Source: CAD feature listing. Evaluate the final solid. Frame: model axes, mm. Face numbers are marked on the shaded views. A direction names the side the tool comes from. Coordinates: 2 decimals unless noted, no trailing zeros. Loops run counter-clockwise (first coordinate to the right, second up) from the corner with the lowest first, then second, coordinate; pieces in that order, holes last. Notation, with made-up numbers: (2, 64.25) -> (57, 64.25) arc R16 ccw to (57, 83.25) -> close; hole circle Ø7 at (63.25, 50.5). An arc over 180 degrees is marked (long way). Answer as CSV lines item,"result".
from build123d import *

# Parameters (mm, degrees)
SCHIZZO1_R                   = 35
ESTRUSIONE_ESTRUSIONE1_DEPTH = 20
SCHIZZO2_R                   = 15
ESTRUSIONE_ESTRUSIONE2_DEPTH = 30
RACCORDO1_R                  = 20


with BuildPart() as part:
    # Schizzo1 → Estrusione-Estrusione1 (new body)
    with BuildSketch(Plane(origin=(0, 0, 0), x_dir=(1, 0, 0), z_dir=(0, 1, 0))):
        with Locations(Location((0, 0, 0), (0, 0, 270))):
            Circle(SCHIZZO1_R)
    extrude(amount=ESTRUSIONE_ESTRUSIONE1_DEPTH)

    # Schizzo2 → Estrusione-Estrusione2 (add)
    with BuildSketch(Plane(origin=(0, 20, 0), x_dir=(1, 0, 0), z_dir=(0, 1, 0))):
        with Locations(Location((0, 0, 0), (0, 0, 270))):
            Circle(SCHIZZO2_R)
    extrude(amount=ESTRUSIONE_ESTRUSIONE2_DEPTH)

    # Raccordo1
    raccordo1_edges = [part.edges().sort_by_distance(p)[0] for p in [
        (0, 20, -15),
    ]]
    fillet(raccordo1_edges, radius=RACCORDO1_R - 0.0001)  # a hair under: the kernel refuses the full size

    # Smusso1: read off the stored shape, not the designer's step
    # Smusso1 outline → Smusso1 (revolve, cut)
    with BuildSketch(Plane.XY):
        Polygon((35, 21.143819168), (28.333333333, 21.143819168), (35, 11.715728753), align=None)
    revolve(axis=Axis((0, 0, 0), (0, 1, 0)), mode=Mode.SUBTRACT)


solid = part.part
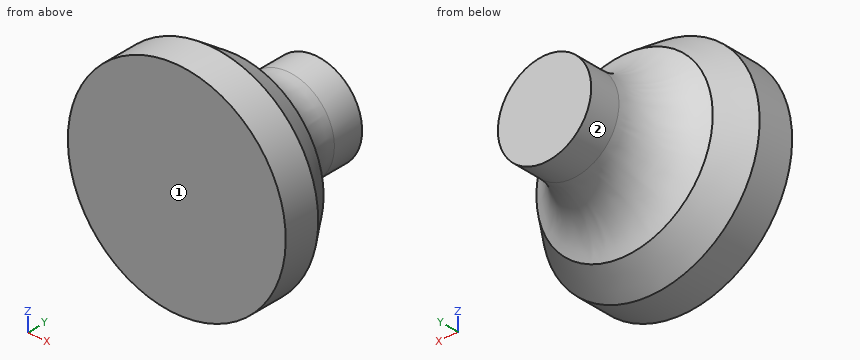
(1) Cut plane A-A (x = 0). Return the cut outline in (y, z).
Computed values:
outline,"(0, -35) -> (11.72, -35) -> (21.14, -28.33) arc R20 cw to (40, -15) -> (50, -15) -> (50, 15) -> (40, 15) arc R20 cw to (21.14, 28.33) -> (11.72, 35) -> (0, 35) -> close"
(2) Access query for the marked faces 1 and 2. Directions: +Z, -Z, +X, -X, +Y, -Y. A direction counts if a zero-diameter tool reaches every point of the face in a straight line with its end or side. Return the directions, or none.
Computed values:
face 1,"+Z, -Z, +X, -X, -Y"
face 2,"+Y"
(3) Cut plane B-B (z = 0). Return the cut outline in (x, y).
Computed values:
outline,"(-35, 0) -> (35, 0) -> (35, 11.72) -> (28.33, 21.14) arc R20 cw to (15, 40) -> (15, 50) -> (-15, 50) -> (-15, 40) arc R20 cw to (-28.33, 21.14) -> (-35, 11.72) -> close"
(4) Pin query (flat end, axial travel): pin 1 Ø2 at (x, y) = (2.5, 13) entering from -Z; pin 2 Ø3 at (x, y) = (-1.5, 16) entering from -Z; pin 3 Ø3 at (y, z) = (5, -18) entering from +X. Return the tip coordinate at first contact, or that it passes through.
Computed values:
pin 1,"z = -34.71"
pin 2,"z = -33"
pin 3,"x = 30.87"
(5) Cut plane D-D (y = 22.5). Return the cut outline in (x, z), then the cut area to 3 significant figures.
Computed values:
outline,"circle Ø50.63 at (0, 0)"
area,"2,010 mm^2"
(6) Cut plane C-C (y = 3.5). Return the cut outline in (x, z), then the cut area to 3 significant figures.
Computed values:
outline,"circle Ø70 at (0, 0)"
area,"3,850 mm^2"
(7) Material intervals for L1, parallel to X at y = 4.5, z = -1; L2, parallel to X at y = 14, z = -21; L3, parallel to Y at x = -21.5, z = 11, sorted ascending. Write a range as [from, to].
Computed values:
L1,"[-34.99, 34.99]"
L2,"[-25.95, 25.95]"
L3,"[0, 23.2]"
